Model file for the job. Use its own axes, mm. A direction names the side the tool comes from. Round coordinates to 2 decimals unless told otherwise and drop trailing zeros. Order: outer loops, then holes, each group sorted by start corner. A loop starts at its lowest first (then second) coordinate and runs counter-clockwise, first axis right, second up. Notation, with made-up numbers: (-5, -38.75) - (1, -38.75) arc R23 cw to (1, -30.75) - close; hole circle Ø5 at (-1, 24.5). An arc over 180 degrees is marked (long way). Write item = value, one per line.
```python
from build123d import *

# Parameters (mm, degrees)
F2_DEPTH = 7
F3_W     = 12.1
F3_H     = 1
F4_DEPTH = 1
F6_DEPTH = 7
F7_DEPTH = 25
F8_R     = 2


with BuildPart() as f2:
    # F1 (on face) → F2 (new body)
    with BuildSketch(Plane.XY):
        Polygon((-6.05, 2.5), (0, 2.5), (0, 4.5), (-7.55, 4.5), (-7.55, -4), (-7.3, -4), (-5.3, -3.25), (-5.3, -2.5), (-6.05, -2.5), align=None)
        Polygon((0, 4.5), (0, 2.5), (6.05, 2.5), (6.05, -2.5), (5.3, -2.5), (5.3, -3.25), (7.3, -4), (7.55, -4), (7.55, 4.5), align=None)
    extrude(amount=F2_DEPTH)

    # F3 (on face) → F4 (join)
    with BuildSketch(Plane.XZ.offset(-2.5)):
        with Locations((0, 3.5)):
            Rectangle(F3_W, F3_H)
    extrude(amount=F4_DEPTH)

    # F5 (on Top) → F6 (join)
    with BuildSketch(Plane.XY):
        Polygon((-10.55, 2.5), (-7.55, 2.5), (-7.55, 4.5), (0, 4.5), (0, 12.5), (-10.55, 12.5), align=None)
        Polygon((0, 12.5), (0, 4.5), (7.55, 4.5), (7.55, 2.5), (10.55, 2.5), (10.55, 12.5), align=None)
    extrude(amount=F6_DEPTH)

    # F5 (on Top) → F7 (join)
    with BuildSketch(Plane.XY):
        Polygon((-7.55, -7.5960563503), (-7.55, -5.5960563503), (-10.55, -5.5960563503), (-10.55, 2.5), (-10.55, 12.5), (0, 12.5), (0, 14.5), (-12.55, 14.5), (-12.55, -7.5960563503), align=None)
        Polygon((0, 14.5), (0, 12.5), (10.55, 12.5), (10.55, 2.5), (10.55, -5.5960563503), (7.55, -5.5960563503), (7.55, -7.5960563503), (12.55, -7.5960563503), (12.55, 14.5), align=None)
    extrude(amount=F7_DEPTH)

    # F8
    f8_edges = [f2.edges().sort_by_distance(p)[0] for p in [
        (12.55, -7.596056, 12.5),
        (10.55, -5.596056, 12.5),
        (-12.55, -7.596056, 12.5),
        (-12.55, 14.5, 12.5),
        (12.55, 14.5, 12.5),
        (-10.55, -5.596056, 12.5),
        (-10.55, 12.5, 16),
        (10.55, 12.5, 16),
    ]]
    fillet(f8_edges, radius=F8_R)


solid = f2.part
```
1) Cut at C-C (y = 5.25). Write the cut outline in (x, z), and give its area (3 significant figures).
Conclusion:
outline = (-12.55, 0) - (12.55, 0) - (12.55, 25) - (10.55, 25) - (10.55, 7) - (-10.55, 7) - (-10.55, 25) - (-12.55, 25) - close
area = 248 mm^2
2) 3-axis set-ups, long thin cutter, end or side, ignore diameter. For faces 4 (the face through (0, 6, 7)), 5 (the face through (-9, 2.5, 3)), 6 (the face through (-7.55, -7, 12)), 7 (the face through (11.949, -7.026, 12.675)): which of +Z, -Z, +X, -X, +Y, -Y reach the whole face in a straight line?
Conclusion:
face_4 = +Z
face_5 = +Z, -Z
face_6 = +Z, -Z, -Y
face_7 = +Z, -Z, +X, -Y
3) Cut at B-B (z = 23). Write the cut outline in (x, y).
Conclusion:
outline = (-12.55, -5.6) arc R2 ccw to (-10.55, -7.6) - (-7.55, -7.6) - (-7.55, -5.6) - (-8.55, -5.6) arc R2 cw to (-10.55, -3.6) - (-10.55, 10.5) arc R2 cw to (-8.55, 12.5) - (8.55, 12.5) arc R2 cw to (10.55, 10.5) - (10.55, -3.6) arc R2 cw to (8.55, -5.6) - (7.55, -5.6) - (7.55, -7.6) - (10.55, -7.6) arc R2 ccw to (12.55, -5.6) - (12.55, 12.5) arc R2 ccw to (10.55, 14.5) - (-10.55, 14.5) arc R2 ccw to (-12.55, 12.5) - close
4) Cut at D-D (x = -4.5). Write the cut outline in (y, z), and give its area (3 significant figures).
Conclusion:
outline = (1.5, 3) - (2.5, 3) - (2.5, 0) - (14.5, 0) - (14.5, 25) - (12.5, 25) - (12.5, 7) - (2.5, 7) - (2.5, 4) - (1.5, 4) - close
area = 121 mm^2
5) Flat gauge pins, fed straight in: pin 1 Ø1 at (y, z) = (-7, 8) entering from -X; pin 2 Ø8 at (x, y) = (2, 1) entering from +Z; pin 3 Ø0.6 at (y, z) = (-7, 7) entering from +X; pin 4 Ø2 at (x, y) = (9, 5) entering from -Z. Where does each tip first touch, or does it go through?
Conclusion:
pin_1 = -12.33
pin_2 = 7
pin_3 = 12.22
pin_4 = 0
6) Cut at A-A (y = -1.75). Write the cut outline in (x, z).
Conclusion:
outline = (-12.55, 0) - (-10.55, 0) - (-10.55, 25) - (-12.55, 25) - close; (-7.55, 0) - (-6.05, 0) - (-6.05, 7) - (-7.55, 7) - close; (6.05, 0) - (7.55, 0) - (7.55, 7) - (6.05, 7) - close; (10.55, 0) - (12.55, 0) - (12.55, 25) - (10.55, 25) - close
7) Mould opens along X. For faces 1 (the face through (-8, -5.596, 12)), 2 (the face through (12.55, 3, 12)), 3 (the face through (-12.55, 4, 12)) say: +X half, -X half, draft (parallel to the pull), parting line (faces both ways), or undercut.
Conclusion:
face_1 = undercut
face_2 = +X half
face_3 = -X half
8) Wall check: line 1 along X through (y, z) = (4.75, 8); line 2 along X through (y, z) = (1.5, 5.5); line 3 along Y through (x, z) = (-8, 10.75). Give the ranges that are in metal, low to high.
Conclusion:
line_1 = -12.55 to -10.55, 10.55 to 12.55
line_2 = -12.55 to -10.55, -7.55 to -6.05, 6.05 to 7.55, 10.55 to 12.55
line_3 = -7.6 to -5.6, 12.5 to 14.5
